from build123d import *

# Parameters (mm, degrees)
SKETCH1_R           = 1
BOSS_EXTRUDE1_DEPTH = 2


with BuildPart() as part:
    # Sketch1 → Boss-Extrude1 (new body)
    with BuildSketch(Plane.XY):
        with BuildLine():
            Line((-15.75, -7), (-15.75, -11))
            Line((-15.75, -11), (-7.75, -11))
            Line((-7.75, -11), (-7.75, -7))
            Line((-7.75, -7), (7.75, -7))
            Line((7.75, -7), (7.75, -11))
            Line((7.75, -11), (15.75, -11))
            Line((15.75, -11), (15.75, -7))
            Line((15.75, -7), (15.75, -1))
            ThreePointArc((15.75, -1), (14.578427125, 1.828427125), (11.75, 3))
            Line((11.75, 3), (-11.75, 3))
            ThreePointArc((-11.75, 3), (-14.578427125, 1.828427125), (-15.75, -1))
            Line((-15.75, -1), (-15.75, -7))
        make_face()
        with Locations((-11.75, 0)):
            Circle(SKETCH1_R, mode=Mode.SUBTRACT)
        with Locations((11.75, 0)):
            Circle(SKETCH1_R, mode=Mode.SUBTRACT)
    extrude(amount=BOSS_EXTRUDE1_DEPTH)


solid = part.part
Design review of the part built by this model. Coordinates are the model's own, in mm. A direction names the side the tool comes from. Give positions to 0.01 mm unless a question says otherwise; leave off trailing zeros. Loops run counter-clockwise (first coordinate to the right, second up) from the corner with the lowest first, then second, coordinate; pieces in that order, holes last. Notation, with made-up numbers: (67, 60) -> (90, 60) arc R17 cw to (90, 73) -> close; hole circle Ø8 at (20, -18). An arc over 180 degrees is marked (long way). One line per question, with ' | ' between items. Start each with the question number.
(1) For line 1 (Y direction, x = -11.75, z = 1.5); line 2 (Y direction, x = -6, z = 0.35); line 3 (X direction, y = -7.5, z = 0.85), list the stretches that pass through material, from the lowest coordinate up.
(2) For faces 4 (the face through (0, 3, 1)), 5 (the face through (0, -7, 1)), list the 3-axis set-ups (+Z, -Z, +X, -X, +Y, -Y) from which the entire face can be reached by the end or side of a thin tool; tool diameter is ignored.
(3) Draft analysis for pull direction X (two halves, no side actions). For faces 1 (the face through (-12, -11, 1)), 2 (the face through (15.75, -6, 1)), 3 (the face through (10.75, 0.04, 0.99)), state which applies: +X half, -X half, draft (parallel to the pull), parting line (faces both ways), or undercut.
(4) We need section D-D (x = 6.5). State the section outline as (y, z) points.
(5) We need section C-C (y = 0). State the section outline as (x, z) points, and give its area (3 significant figures).
(6) We need section A-A (z = 0.55). State the section outline as (x, y) points, and give its area (3 significant figures).
(7) We need section B-B (y = -9.25). State the section outline as (x, z) points.
The answers:
1) line 1: y = -11 to -1, 1 to 3 | line 2: y = -7 to 3 | line 3: x = -15.75 to -7.75, 7.75 to 15.75
2) face 4: +Z, -Z, +X, -X, +Y | face 5: +Z, -Z, -Y
3) face 1: draft | face 2: +X half | face 3: undercut
4) outline: (-7, 0) -> (3, 0) -> (3, 2) -> (-7, 2) -> close
5) outline: (-15.62, 0) -> (-12.75, 0) -> (-12.75, 2) -> (-15.62, 2) -> close; (-10.75, 0) -> (10.75, 0) -> (10.75, 2) -> (-10.75, 2) -> close; (12.75, 0) -> (15.62, 0) -> (15.62, 2) -> (12.75, 2) -> close | area: 54.5 mm^2
6) outline: (-15.75, -11) -> (-7.75, -11) -> (-7.75, -7) -> (7.75, -7) -> (7.75, -11) -> (15.75, -11) -> (15.75, -1) arc R4 ccw to (11.75, 3) -> (-11.75, 3) arc R4 ccw to (-15.75, -1) -> close; hole circle Ø2 at (-11.75, 0); hole circle Ø2 at (11.75, 0) | area: 366 mm^2
7) outline: (-15.75, 0) -> (-7.75, 0) -> (-7.75, 2) -> (-15.75, 2) -> close; (7.75, 0) -> (15.75, 0) -> (15.75, 2) -> (7.75, 2) -> close
